Here's how the part is built. I have some questions about the finished solid (model axes, mm). Round coordinates to 2 decimals unless told otherwise and drop trailing zeros. Loops run counter-clockwise (first coordinate to the right, second up) from the corner with the lowest first, then second, coordinate; pieces in that order, holes last. Notation, with made-up numbers: M 66,55 L 101,55 A27 ccw 101,93 Z; hole C 25.5,5 d6. An arc over 180 degrees is marked long. Use a Markdown table: item, result.
```python
from build123d import *

# Parameters (mm, degrees)
SKETCH89_R          = 0.76
BOSS_EXTRUDE1_DEPTH = 2.5
SKETCH91_W          = 4.4
SKETCH91_H          = 7.5
CUT_EXTRUDE1_DEPTH  = 1.5


with BuildPart() as part:
    # Sketch89 → Boss-Extrude1 (new body)
    with BuildSketch(Plane(origin=(0, 33.039348741, 0), x_dir=(1, 0, 0), z_dir=(0, 1, 0))):
        with BuildLine():
            Line((-2.2, 31.284010223), (2.2, 31.284010223))
            ThreePointArc((2.2, 31.284010223), (33.484010223, 0), (2.2, -31.284010223))
            Line((2.2, -31.284010223), (-2.2, -31.284010223))
            ThreePointArc((-2.2, -31.284010223), (-33.484010223, 0), (-2.2, 31.284010223))
        make_face()
        with Locations(Location((0, 28, 0), (0, 0, 270))):
            Circle(SKETCH89_R, mode=Mode.SUBTRACT)
        with Locations(Location((0, -28, 0), (0, 0, 270))):
            Circle(SKETCH89_R, mode=Mode.SUBTRACT)
        with BuildLine():
            ThreePointArc((-5.285684122, 23.410714286), (0, 21), (5.285684122, 23.410714286))
            ThreePointArc((5.285684122, 23.410714286), (24, 0), (5.285684122, -23.410714286))
            ThreePointArc((5.285684122, -23.410714286), (0, -21), (-5.285684122, -23.410714286))
            ThreePointArc((-5.285684122, -23.410714286), (-24, 0), (-5.285684122, 23.410714286))
        make_face(mode=Mode.SUBTRACT)
    extrude(amount=BOSS_EXTRUDE1_DEPTH)

    # Sketch91 → Cut-Extrude1 (cut)
    with BuildSketch(Plane.XZ.offset(-33.039348741)):
        with Locations((0, 27.534010223)):
            Rectangle(SKETCH91_W, SKETCH91_H)
        with Locations((0, -27.534010223)):
            Rectangle(SKETCH91_W, SKETCH91_H)
    extrude(amount=-CUT_EXTRUDE1_DEPTH, mode=Mode.SUBTRACT)


solid = part.part
```
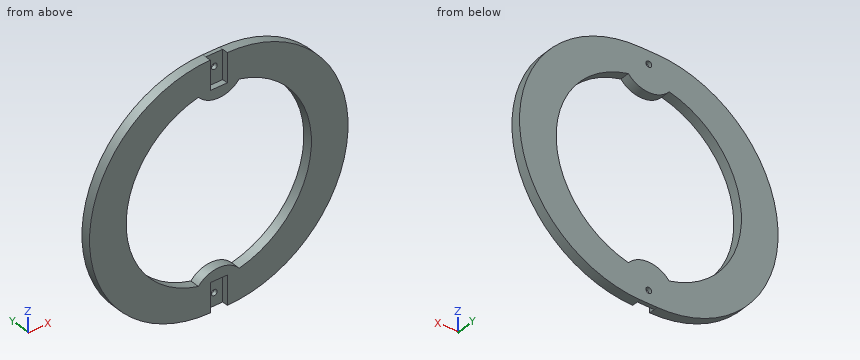
Q1. Imagine slicing it at B-B, the plane z = 0. Please give me the cut outline in (x, y), then the cut area to 3 significant figures.
Return value:
| item | result |
|---|---|
| outline | M -33.48,33.04 L -24,33.04 L -24,35.54 L -33.48,35.54 Z; M 24,33.04 L 33.48,33.04 L 33.48,35.54 L 24,35.54 Z |
| area | 47.4 mm^2 |
Q2. I need wall thicknesses on line 1 (Z direction, x = -18, y = 33.5); line 2 (X direction, y = 34.8, z = 8.5); line 3 (X direction, y = 35, z = -28). Which ranges of each line are inside material? Lowest first, please. Write a range as from..to.
Return value:
| item | result |
|---|---|
| line 1 | z = -27..-15.87, 15.87..27 |
| line 2 | x = -32.31..-22.44, 22.44..32.31 |
| line 3 | x = -16.15..-0.76, 0.76..16.15 |
Q3. Imagine slicing it at A-A, the plane x = 0. Please give me the cut outline in (y, z).
Return value:
| item | result |
|---|---|
| outline | M 33.04,-23.78 L 34.54,-23.78 L 34.54,-27.24 L 35.54,-27.24 L 35.54,-21 L 33.04,-21 Z; M 33.04,21 L 35.54,21 L 35.54,27.24 L 34.54,27.24 L 34.54,23.78 L 33.04,23.78 Z; M 34.54,-31.28 L 35.54,-31.28 L 35.54,-28.76 L 34.54,-28.76 Z; M 34.54,28.76 L 35.54,28.76 L 35.54,31.28 L 34.54,31.28 Z |
Q4. Will these pins go through, and if not, where does the flat tip stop? P1, Ø1.5, axis at y = 33.5, z = -1, coming from the -X side; P2, Ø1, axis at y = 33.5, z = 12.5, coming from the -X side; P3, Ø1.2, axis at y = 34, z = -26, coming from the +X side.
Return value:
| item | result |
|---|---|
| P1 | stops at x = -33.48 |
| P2 | stops at x = -31.09 |
| P3 | stops at x = 20.46 |
Q5. Imagine slicing it at C-C, the plane y = 33.6. Please give me the cut outline in (x, z), then the cut area to 3 significant figures.
Return value:
| item | result |
|---|---|
| outline | M -2.2,-31.28 L -2.2,-23.78 L 2.2,-23.78 L 2.2,-31.28 A31.28 ccw 2.2,31.28 L 2.2,23.78 L -2.2,23.78 L -2.2,31.28 A31.28 ccw Z; hole M -5.29,-23.41 A7 cw 5.29,-23.41 A24 ccw 5.29,23.41 A7 cw -5.29,23.41 A24 ccw Z |
| area | 1,520 mm^2 |
Q6. Imagine slicing it at D-D, the plane z = 10.5. Please give me the cut outline in (x, y), then the cut area to 3 significant figures.
Return value:
| item | result |
|---|---|
| outline | M -31.67,33.04 L -21.58,33.04 L -21.58,35.54 L -31.67,35.54 Z; M 21.58,33.04 L 31.67,33.04 L 31.67,35.54 L 21.58,35.54 Z |
| area | 50.4 mm^2 |
